Geometry: final body of the model. Coordinates: model frame, mm. A direction names the side the tool comes from. Round coordinates to 2 decimals unless told otherwise and drop trailing zeros. Write each loop counter-clockwise with the first axis right and the second up, starting at its lowest first coordinate (ties: lowest second). Pieces come first, ordered by that corner, then holes. Notation, with made-up numbers: M 1.25,-35 L 23.25,-35 A13 ccw 23.25,-20 Z; hole C 6,-6 d2. An arc over 180 degrees is marked long. Use one line per item in the form item = value. Start each with the question number.
from build123d import *

# Parameters (mm, degrees)
SKETCH1_R           = 19
SKETCH1_R_2         = 13
BOSS_EXTRUDE1_DEPTH = 55
SKETCH2_W           = 8
SKETCH2_H           = 6
CUT_EXTRUDE3_DEPTH  = 24
FILLET5_R           = 4
FILLET6_R           = 4
SKETCH3_R           = 1.5
CUT_EXTRUDE11_DEPTH = 68.904344566


with BuildPart() as part:
    # Sketch1 → Boss-Extrude1 (new body)
    with BuildSketch(Plane.XY):
        Circle(SKETCH1_R)
        Circle(SKETCH1_R_2, mode=Mode.SUBTRACT)
    extrude(amount=BOSS_EXTRUDE1_DEPTH)

    # Sketch2 → Cut-Extrude3 (cut)
    with BuildSketch(Plane.XY.offset(55)):
        with Locations((0, 13)):
            Rectangle(SKETCH2_W, SKETCH2_H)
    extrude(amount=-CUT_EXTRUDE3_DEPTH, mode=Mode.SUBTRACT)

    # Fillet5
    fillet5_edges = [part.edges().sort_by_distance(p)[0] for p in [
        (4, 14.184658438, 31),
    ]]
    fillet(fillet5_edges, radius=FILLET5_R)

    # Fillet6
    fillet6_edges = [part.edges().sort_by_distance(p)[0] for p in [
        (-4, 14.184658438, 31),
    ]]
    fillet(fillet6_edges, radius=FILLET6_R - 0.0001)  # a hair under: the kernel refuses the full size

    # Sketch3 → Cut-Extrude11 (cut, through all)
    with BuildSketch(Plane(origin=(0, 16, 0), x_dir=(-1, 0, 0), z_dir=(0, -1, 0))):
        with Locations(Location((0, -49, 0), (0, 0, 90))):
            Circle(SKETCH3_R)
    extrude(amount=-CUT_EXTRUDE11_DEPTH, mode=Mode.SUBTRACT)


solid = part.part
1. Section query B-B (x = -6). Return loops of the section in (y, z).
2. Pull-direction query (Y, two-part tool) for faces 4 (the face through (8.767, -16.856, 27.115)), 5 (the face through (-4.5, -12.4, 55)), 6 (the face through (-2.797, 14.21, 32.141)), 7 (the face through (-2.82, -12.69, 27.12)); classes: released by +Y, released by -Y, zero draft, split by the parting line, or undercut.
3. Ray query, probe 1 along Z at (x, y) = (0, 17.2); probe 2 along Y at (x, z) = (0, 34); probe 3 along Y at (x, z) = (0, 14). Return the intervals inside material, ascending.
4. Section query A-A (y = 0). Return loops of the section in (x, z), then the cut area to 3 significant figures.
5. Section query C-C (z = 39). Return loops of the section in (x, y), then the cut area to 3 significant figures.
6. Set-up query: faces 1 (the face through (-4.5, -12.4, 0)), 2 (the face through (0, 16, 43)), 3 (the face through (0.07, 17.48, 50.5)). Return all of +Z, -Z, +X, -X, +Y, -Y with unobstructed straight access to the full face (end or side cutting, diameter ignored); none if empty.
7. Contact query for flat-ended pins moving along their axis: pin 1 (10 mm diameter, centred on x = 4.5, z = 36, fed in from -Y); pin 2 (12 mm diameter, centred on x = -9, z = 47, fed in from -Y); pin 3 (1.1 mm diameter, centred on y = 13.5, z = 48.5, fed in from -X). Output: stop coordinate, or through.
8. Section query D-D (z = 49). Return loops of the section in (x, y), then the cut area to 3 significant figures.
Checks:
q1.outline = M -18.03,0 L -11.53,0 L -11.53,55 L -18.03,55 Z; M 11.53,0 L 18.03,0 L 18.03,55 L 11.53,55 Z
q2.face_4 = split by the parting line
q2.face_5 = zero draft
q2.face_6 = undercut
q2.face_7 = undercut
q3.probe_1 = 0 to 47.5, 50.5 to 55
q3.probe_2 = -19 to -13, 16 to 19
q3.probe_3 = -19 to -13, 13 to 19
q4.outline = M -19,0 L -13,0 L -13,55 L -19,55 Z; M 13,0 L 19,0 L 19,55 L 13,55 Z
q4.area = 660 mm^2
q5.outline = C 0,0 d38; hole M -4,12.37 A13 ccw long 4,12.37 L 4,16 L -4,16 Z
q5.area = 578 mm^2
q6.face_1 = -Z, +X, -X, +Y, -Y
q6.face_2 = +Z
q6.face_3 = +Y
q7.pin_1 = -19
q7.pin_2 = -18.76
q7.pin_3 = -13.9
q8.outline = M -4,12.37 L -4,16 L -1.5,16 L -1.5,18.94 A19 ccw long 1.5,18.94 L 1.5,16 L 4,16 L 4,12.37 A13 cw long Z
q8.area = 569 mm^2
